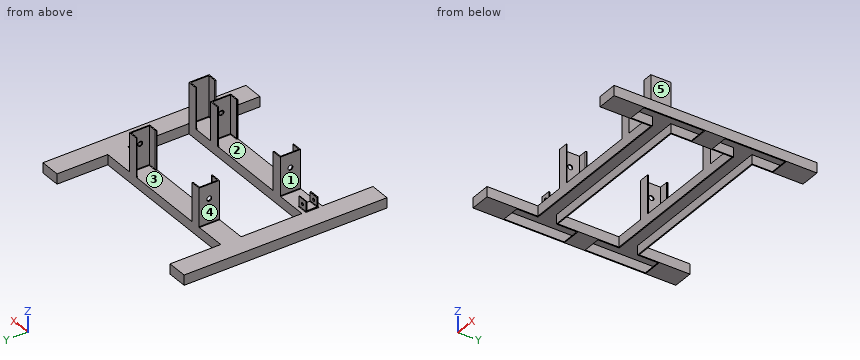
```python
from build123d import *

# Parameters (mm, degrees)
F0_W      = 805
F0_H      = 100
F0_W_2    = 100
F0_H_2    = 150
F1_DEPTH  = 50
F2_T      = -5
F3_DEPTH  = 5
F5_DEPTH  = 190
F7_D      = 24
F11_W     = 50
F11_H     = 50
F12_DEPTH = 5
F11_H_2   = 5
F13_DEPTH = 50
F14_DEPTH = 200
F16_D     = 14
F17_R     = 2.5


with BuildPart() as f1:
    # F0 (on Top) → F1 (new body)
    with BuildSketch(Plane.XY):
        with Locations((0, 200)):
            Rectangle(F0_W, F0_H)
        Polygon((-402.5, 50), (-402.5, 150), (-402.5, 250), (-402.5, 350), (-502.5, 350), (-502.5, 50), align=None)
        Polygon((402.5, 250), (402.5, 150), (402.5, 50), (502.5, 50), (502.5, 350), (402.5, 350), align=None)
        Polygon((-402.5, 0), (-402.5, 50), (-502.5, 50), (-502.5, 0), (-502.5, -50), (-402.5, -50), align=None)
        Polygon((502.5, 50), (402.5, 50), (402.5, 0), (402.5, -50), (502.5, -50), (502.5, 0), align=None)
        with Locations((-452.5, 425)):
            Rectangle(F0_W_2, F0_H_2)
        with Locations((452.5, 425)):
            Rectangle(F0_W_2, F0_H_2)
        Polygon((-402.5, -150), (-402.5, -50), (-502.5, -50), (-502.5, -350), (-402.5, -350), (-402.5, -250), align=None)
        Polygon((502.5, -50), (402.5, -50), (402.5, -150), (402.5, -250), (402.5, -350), (502.5, -350), align=None)
        with Locations((0, -200)):
            Rectangle(F0_W, F0_H)
        with Locations((-452.5, -425)):
            Rectangle(F0_W_2, F0_H_2)
        with Locations((452.5, -425)):
            Rectangle(F0_W_2, F0_H_2)
    extrude(amount=F1_DEPTH)

    # F2
    f2_openings = [f1.faces().sort_by_distance(p)[0] for p in [
        (0, 164.177535, 0),
    ]]
    offset(amount=F2_T, openings=f2_openings, kind=Kind.INTERSECTION)

    # F0 (on Top) → F3 (join)
    with BuildSketch(Plane.XY):
        with Locations((-452.5, -425)):
            Rectangle(F0_W_2, F0_H_2)
        Polygon((-402.5, 0), (-402.5, 50), (-502.5, 50), (-502.5, 0), (-502.5, -50), (-402.5, -50), align=None)
        with Locations((-452.5, 425)):
            Rectangle(F0_W_2, F0_H_2)
        with Locations((452.5, -425)):
            Rectangle(F0_W_2, F0_H_2)
        Polygon((502.5, 50), (402.5, 50), (402.5, 0), (402.5, -50), (502.5, -50), (502.5, 0), align=None)
        with Locations((452.5, 425)):
            Rectangle(F0_W_2, F0_H_2)
    extrude(amount=F3_DEPTH)


with BuildPart() as f5:
    # F4 (on face) → F5 (new body)
    with BuildSketch(Plane.XY.offset(50)):
        with BuildLine():
            Line((198, -250), (248, -250))
            Line((248, -250), (248, -150))
            Line((248, -150), (198, -150))
            Line((198, -150), (198, -150.9999952316))
            ThreePointArc((198, -150.9999952316), (199.1715728753, -153.8284223564), (202, -154.9999952316))
            Line((202, -154.9999952316), (243.0000047684, -154.9999952316))
            Line((243.0000047684, -154.9999952316), (243.0000047684, -245.0000047684))
            Line((243.0000047684, -245.0000047684), (202, -245.0000047684))
            ThreePointArc((202, -245.0000047684), (199.1715728753, -246.1715776436), (198, -249.0000047684))
            Line((198, -249.0000047684), (198, -250))
        make_face()
    extrude(amount=F5_DEPTH)

    # F7 (through all)
    with Locations(Plane.YZ.offset(248)):
        with Locations((-200, 170)):
            Hole(F7_D / 2)


with BuildPart() as f8_1:
    # F8: instance of F5
    add(f5.part.mirror(Plane.YZ))


with BuildPart() as f9_1:
    # F9: instance of F5
    add(f5.part.mirror(Plane.XZ))


with BuildPart() as f9_2:
    # F9: instance of F8_1
    add(f8_1.part.mirror(Plane.XZ))


with BuildPart() as f8_1_1:
    add(f8_1.part)

    # F10: union F9_2, F5, F9_1, F1
    add(f9_2.part)
    add(f5.part)
    add(f9_1.part)
    add(f1.part)

    # F11 (on face) → F12 (join)
    with BuildSketch(Plane.XY.offset(50)):
        with Locations((-377.5, -200)):
            Rectangle(F11_W, F11_H)
    extrude(amount=F12_DEPTH)

    # F11 (on face) → F13 (join)
    with BuildSketch(Plane.XY.offset(50)):
        with Locations((-377.5, -227.5)):
            Rectangle(F11_W, F11_H_2)
        with Locations((-377.5, -172.5)):
            Rectangle(F11_W, F11_H_2)
    extrude(amount=F13_DEPTH)

    # F11 (on face) → F14 (join)
    with BuildSketch(Plane.XY.offset(50)):
        with BuildLine():
            Line((402.5, -250), (402.5, -150))
            Line((402.5, -150), (352.5, -150))
            Line((352.5, -150), (352.5, -151.0000011921))
            ThreePointArc((352.5, -151.0000011921), (353.6715728753, -153.8284283168), (356.5, -155.0000011921))
            Line((356.5, -155.0000011921), (397.4999988079, -155.0000011921))
            Line((397.4999988079, -155.0000011921), (397.4999988079, -244.9999988079))
            Line((397.4999988079, -244.9999988079), (356.5, -244.9999988079))
            ThreePointArc((356.5, -244.9999988079), (353.6715728753, -246.1715716832), (352.5, -248.9999988079))
            Line((352.5, -248.9999988079), (352.5, -250))
            Line((352.5, -250), (402.5, -250))
        make_face()
    extrude(amount=F14_DEPTH)

    # F16 (through all)
    with Locations(Plane.XZ.offset(230)):
        with Locations((-377.5, 75)):
            Hole(F16_D / 2)

    # F17
    f17_edges = [f8_1_1.edges().sort_by_distance(p)[0] for p in [
        (-377.5, -175, 55),
        (-377.5, -225, 55),
        (-377.5, -225, 100),
        (-377.5, -175, 100),
        (-377.5, -230, 50),
        (-402.5, -200, 50),
        (-377.5, -170, 50),
        (-352.5, -200, 50),
        (-248, -200, 50),
        (-248, 200, 50),
        (243.000005, -200, 50),
        (222.500002, -154.999995, 50),
        (199.171573, -153.828422, 50),
        (222.500002, -245.000005, 50),
        (199.171573, -246.171578, 50),
        (222.500002, 245.000005, 50),
        (199.171573, 246.171578, 50),
        (243.000005, 200, 50),
        (222.500002, 154.999995, 50),
        (199.171573, 153.828422, 50),
        (248, 200, 50),
        (248, -200, 50),
        (376.999999, -155.000001, 50),
        (353.671573, -153.828428, 50),
        (397.499999, -200, 50),
        (376.999999, -244.999999, 50),
        (353.671573, -246.171572, 50),
        (402.5, -200, 50),
        (-222.500002, 154.999995, 50),
        (-199.171573, 153.828422, 50),
        (-243.000005, 200, 50),
        (-222.500002, 245.000005, 50),
        (-199.171573, 246.171578, 50),
        (-222.500002, -154.999995, 50),
        (-199.171573, -153.828422, 50),
        (-222.500002, -245.000005, 50),
        (-199.171573, -246.171578, 50),
        (-243.000005, -200, 50),
    ]]
    fillet(f17_edges, radius=F17_R)


solid = f8_1_1.part
```
Work out the finished part from the listing and answer in its coordinate system (mm). Face numbers are marked on the shaded views. A direction names the side the tool comes from. Coordinates: 2 decimals unless noted, no trailing zeros. Loops run counter-clockwise (first coordinate to the right, second up) from the corner with the lowest first, then second, coordinate; pieces in that order, holes last. Notation, with made-up numbers: (19.5, 21.25) -> (28.5, 21.25) arc R22 cw to (28.5, 49.25) -> close; hole circle Ø9 at (41, 27). An arc over 180 degrees is marked (long way). Answer as CSV lines item,"result".
Q1. The part is cut by section C-C on z = 25.5. State how many separate pieces and enclosed holes the cut face has, and give its area (3 significant figures).
Findings:
separate pieces,"2"
enclosed holes,"2"
area,"36,100 mm²"
Q2. The part is cut by section B-B on x = 11.5. Write down the section's boundary in (y, z).
Findings:
outline,"(-250, 0) -> (-245, 0) -> (-245, 45) -> (-155, 45) -> (-155, 0) -> (-150, 0) -> (-150, 50) -> (-250, 50) -> close; (150, 0) -> (155, 0) -> (155, 45) -> (245, 45) -> (245, 0) -> (250, 0) -> (250, 50) -> (150, 50) -> close"
Q3. Each of these flat-tipped pins is pushed along its axis until it touches: pin 1 (24 mm diameter, centred on y = -211.5, z = 82.5, fed in from -X); pin 2 (2 mm diameter, centred on y = 151.5, z = 148, fed in from +X); pin 3 (10 mm diameter, centred on x = -206, z = 188.5, fed in from +Y). Where does it stop, or does it pass through?
Findings:
pin 1,"stops at x = -248"
pin 2,"stops at x = 248"
pin 3,"stops at y = 250"
Q4. For a pull along Y with two mould halves and no side action, classify the marked faces 1 and 2 as +Y half, -Y half, draft (parallel to the pull), parting line (faces both ways), or undercut.
Findings:
face 1,"draft"
face 2,"undercut"
Q5. Find the intervals of material crossed by probe 1 along X at (y, z) = (-248.5, 76.5); probe 2 along X at (y, z) = (19, 39.5); probe 3 along Y at (x, z) = (434.5, 28), in increasing order.
Findings:
probe 1,"x = -248 to -198.03, 198.03 to 248, 352.53 to 402.5"
probe 2,"x = -502.5 to -497.5, -407.5 to -402.5, 402.5 to 407.5, 497.5 to 502.5"
probe 3,"y = -500 to -495, 495 to 500"
Q6. The part is cut by section D-D on y = 200. Write down the section's boundary in (x, z).
Findings:
outline,"(-502.5, 0) -> (-497.5, 0) -> (-497.5, 45) -> (497.5, 45) -> (497.5, 0) -> (502.5, 0) -> (502.5, 50) -> (250.5, 50) arc R2.5 cw to (248, 52.5) -> (248, 158) -> (243, 158) -> (243, 52.5) arc R2.5 cw to (240.5, 50) -> (-240.5, 50) arc R2.5 cw to (-243, 52.5) -> (-243, 158) -> (-248, 158) -> (-248, 52.5) arc R2.5 cw to (-250.5, 50) -> (-502.5, 50) -> close; (-248, 182) -> (-243, 182) -> (-243, 240) -> (-248, 240) -> close; (243, 182) -> (248, 182) -> (248, 240) -> (243, 240) -> close"
Q7. The part is cut by section A-A on y = -385. Write down the section's boundary in (x, z).
Findings:
outline,"(-502.5, 0) -> (-402.5, 0) -> (-402.5, 50) -> (-502.5, 50) -> close; (402.5, 0) -> (502.5, 0) -> (502.5, 50) -> (402.5, 50) -> close; hole (-497.5, 5) -> (-407.5, 5) -> (-407.5, 45) -> (-497.5, 45) -> close; hole (407.5, 5) -> (497.5, 5) -> (497.5, 45) -> (407.5, 45) -> close"
Q8. A tool of negligible diameter and unlimited length cuts with its end or side. For the marked faces 3, 4 and 5, from which of +Z, -Z, +X, -X, +Y, -Y can it reach the whole face along a straight path? Write none if from no direction.
Findings:
face 3,"+Z"
face 4,"+Z, -X, +Y, -Y"
face 5,"+Z, +X, +Y, -Y"
